Autodesk Inventor part; units mm, degrees
ref_plane "WorkPlane2" through (0, 0, 0) normal (0, 0, 1) x (1, 0, 0)
ref_plane "WorkPlane3" through (0, 0, -7) normal (0, 0, 1) x (1, 0, 0)
ref_plane "YZ Plane" through (0, 0, 0) normal (1, 0, 0) x (0, 1, 0)
ref_plane "WorkPlane2" through (0, 0, 0) normal (0, 0, 1) x (1, 0, 0)
sketch "Sketch1" plane through (0, 0, 0) normal (0, 1, 0) x (-1, 0, 0)
  point P0 (0, 0)
ref_plane "WorkPlane3" through (0, 0, -7) normal (0, 0, 1) x (1, 0, 0)
sketch "Sketch2" plane through (0, 0, 0) normal (0, 1, 0) x (-1, 0, 0)
  line L0 (16.55, -0.7) -> (25.3, -0.7)
  line L1 (16.55, -0.35) -> (16.55, -0.7)
  line L2 (23.3, -0.35) -> (16.55, -0.35)
  line L3 (23.3, 0) -> (23.3, -0.35)
  line L4 (26, 0) -> (23.3, 0)
  line L5 (26, -7) -> (26, 0)
  line L6 (15.2, -7) -> (26, -7)
  line L7 (14.525, -4.0833) -> (15.2, -7)
  line L8 (13.85, -3.5) -> (14.525, -4.0833)
  line L9 (12.5, -1.75) -> (13.85, -3.5)
  line L10 (13.85, -1.05) -> (12.5, -1.75)
  line L11 (16.55, -1.05) -> (13.85, -1.05)
  line L12 (16.55, -1.05) -> (16.55, -6.3)
  line L13 (25.3, -6.3) -> (16.55, -6.3)
  line L14 (25.3, -0.7) -> (25.3, -6.3)
  line L15 (0, -15.959) -> (0, -1.7548) construction
  line L16 (0, -15.959) -> (0, -1.7548)
  line L17 (0, -19.1509) -> (0, 3.1918)
  line L18 (-5.2, 0) -> (31.2, 0)
  dimension "d2" = 7
  dimension "d4" = 0.35
  dimension "d6" = 0.35
  dimension "d8" = 0.35
  dimension "d10" = 0.7
  dimension "d12" = 0.7
  dimension "d14" = 2.7
  dimension "d16" = 2.7
  dimension "d18" = 2.9167
  dimension "d20" = 1.75
  dimension "d22" = 1.35
  dimension "d24" = 0.7
  dimension "d26" = 0.675
  dimension "d28" = 1.35
  dimension "d30" = 0.675
  dimension "msp_d33" = 25
  dimension "msp_d34" = 52
revolve "Revolution1" add sketch "Sketch2" angle 360 about axis through (0, 0, -15.959) along (0, 0, -1)
fillet "Fillet1" radius 0.35 4 edges at (26, 0, 0) (26, 0, -7) (14.525, 0, -4.0833) (16.55, 0, -1.05)
equation "\"d32\" = 0.05 * b"
equation "\"d2\" = b"
equation "\"d4\" = 0.05 * b"
equation "\"d6\" = 0.05 * b"
equation "\"d8\" = 0.05 * b"
equation "\"d10\" = 0.1 * b"
equation "\"d12\" = 0.1 * b"
equation "\"d14\" = 0.1 * dd - 0.1 * Diam"
equation "\"d16\" = 0.1 * dd - 0.1 * Diam"
equation "\"d18\" = 0.416667 * b"
equation "\"d20\" = 0.25 * b"
equation "\"d22\" = 0.05 * dd - 0.05 * Diam"
equation "\"d24\" = 0.1 * b"
equation "\"d26\" = 0.025 * dd - 0.025 * Diam"
equation "\"d28\" = 0.05 * dd - 0.05 * Diam"
equation "\"d30\" = 0.025 * dd - 0.025 * Diam"
equation "\"msp_d33\" = Diam"
equation "\"msp_d34\" = dd"
equation "\"dd\" = 52"
equation "\"Diam\" = 25"
properties part number "IS0 6194/1 - 25x52x7-Type 3" material "Rubber"
Verification items for the finished model (mm, model axes). A direction names the side the tool comes from. Coordinates: 2 decimals unless noted, no trailing zeros.
Item 1: Material ranges on L1, parallel to Z at x = 5, y = 20.5; L2, parallel to Z at x = 20, y = -15; L3, parallel to X at y = -7.5, z = -4.5, recorded low to high.
Filled in:
L1: z = -7 to -6.3, -0.7 to -0.35
L2: z = -7 to -6.3, -0.7 to 0
L3: x = -24.89 to -24.16, -14.75 to -12.55, 12.55 to 14.75, 24.16 to 24.89
Item 2: Access from +Z, -Z, +X, -X, +Y, -Y to the whole of each face (thin tool, end or side, straight path). Record for faces 1 (the face through (3.588, -16.156, -3.884)), 2 (the face through (-13.124, 4.876, -1.05)), 3 (the face through (12.6, 0.6, -1.9)).
Filled in:
face 1: none
face 2: +Z
face 3: -Z
Item 3: Release check for a two-part mould opening along Y. For faces 4 (the face through (-5, 16, -0.35)), 5 (the face through (-11, -11, -7)), 6 (the face through (20.633, 15.821, -3.456)), 7 (the face through (-6.733, -12.945, -4.37)) record: +Y half, -Y half, draft (parallel to the pull), parting line (faces both ways), or undercut.
Filled in:
face 4: undercut
face 5: draft
face 6: parting line
face 7: undercut
Item 4: Depth check by flat-ended pin: pin 1 (5 mm diameter, centred on x = 12, y = 12, fed in from +Z); pin 2 (2 mm diameter, centred on y = 5.5, z = -2.5, fed in from +X); pin 3 (3 mm diameter, centred on x = -11.5, z = -2, fed in from -Y). Enter the tip coordinate at first touch or a pass-through.
Filled in:
pin 1: stops at z = -0.35
pin 2: stops at x = 25.61
pin 3: stops at y = -24
